from build123d import *

# Parameters (mm, degrees)
BOSS_EXTRUDE1_DEPTH = 6.35
CUT_EXTRUDE4_DEPTH  = 6.35
SKETCH3_R           = 3.2639
CUT_EXTRUDE5_DEPTH  = 6.35


with BuildPart() as part:
    # Sketch1 → Boss-Extrude1 (new body)
    with BuildSketch(Plane(origin=(0, 0, 0), x_dir=(0, 0, -1), z_dir=(1, 0, 0))):
        with BuildLine():
            Line((152.4, 0), (152.4, -50.8))
            Line((152.4, -50.8), (203.2, -50.8))
            Line((203.2, -50.8), (203.2, 0))
            ThreePointArc((203.2, 0), (190.945540544, 69.498493124), (155.660230842, 130.614442288))
            Line((155.660230842, 130.614442288), (116.745173131, 97.960831716))
            ThreePointArc((116.745173131, 97.960831716), (143.209155408, 52.123869843), (152.4, 0))
        make_face()
    extrude(amount=BOSS_EXTRUDE1_DEPTH)

    # Sketch2 → Cut-Extrude4 (cut)
    with BuildSketch(Plane(origin=(6.35, 0, 0), x_dir=(0, 0, -1), z_dir=(1, 0, 0))):
        with BuildLine():
            ThreePointArc((134.46138915, 101.323924376), (129.890458655, 101.966326764), (129.248056268, 97.395396268))
            ThreePointArc((129.248056268, 97.395396268), (153.473001896, 51.351348104), (161.8361, 0))
            ThreePointArc((161.8361, 0), (165.1, -3.2639), (168.3639, 0))
            ThreePointArc((168.3639, 0), (159.663469053, 53.422649441), (134.46138915, 101.323924376))
        make_face()
        with BuildLine():
            ThreePointArc((154.746731105, 116.610025965), (150.17580061, 117.252428352), (149.533398223, 112.681497856))
            ThreePointArc((149.533398223, 112.681497856), (177.560422739, 59.410886377), (187.2361, 0))
            ThreePointArc((187.2361, 0), (190.5, -3.2639), (193.7639, 0))
            ThreePointArc((193.7639, 0), (183.750889895, 61.482187713), (154.746731105, 116.610025965))
        make_face()
    extrude(amount=-CUT_EXTRUDE4_DEPTH, mode=Mode.SUBTRACT)

    # Sketch3 → Cut-Extrude5 (cut)
    with BuildSketch(Plane(origin=(6.35, 0, 0), x_dir=(0, 0, -1), z_dir=(1, 0, 0))):
        with Locations((165.1, -38.1)):
            Circle(SKETCH3_R)
        with Locations((190.5, -38.1)):
            Circle(SKETCH3_R)
    extrude(amount=-CUT_EXTRUDE5_DEPTH, mode=Mode.SUBTRACT)

    # Sketch7 → Cut-Revolve1 (revolve, cut)
    with BuildSketch(Plane(origin=(0, 0, 0), x_dir=(1, 0, 0), z_dir=(0, 1, 0))):
        with BuildLine():
            Line((-25.4, 38.1), (-144.027789746, 38.1))
            ThreePointArc((-144.027789746, 38.1), (-25.4, 156.727789746), (93.227789746, 38.1))
            Line((93.227789746, 38.1), (-25.4, 38.1))
        make_face()
    revolve(axis=Axis((-1000, 0, 0), (1, 0, 0)), mode=Mode.SUBTRACT)


solid = part.part
The model under review builds one solid part; all positions refer to its coordinate system, in mm. A direction names the side the tool comes from. Round coordinates to 2 decimals unless told otherwise and drop trailing zeros. Write each loop counter-clockwise with the first axis right and the second up, starting at its lowest first coordinate (ties: lowest second). Pieces come first, ordered by that corner, then holes. Notation, with made-up numbers: M 26,8 L 48,8 A8 cw 48,23 Z; hole C 16.5,-16.5 d8. An arc over 180 degrees is marked long. Use a Markdown table: item, result. Add a question column.
Q1. Insertion check: pin 1 (1.9 mm diameter, centred on x = 2.5, y = -33, fed in from +Z); pin 2 (5 mm diameter, centred on y = 32.5, z = -149, fed in from -X); pin 3 (3 mm diameter, centred on x = 0.5, z = -139, fed in from -Y); pin 4 (1 mm diameter, centred on x = 3, z = -137, fed in from +Y). Each pin has a flat end and moves straight along its axis. Give the tip position at first contact, or say it passes through.
Q2. We need section C-C, the plane z = -183. State the section outline as (x, y) points, plus the area to 3 significant figures.
Q3. We need section A-A, the plane y = -38.1. State the section outline as (x, z) points, plus the area to 3 significant figures.
Q4. To check wall thickness, follow line 1 (Z direction, x = 6, y = 88); line 2 (Z direction, x = 5.5, y = 56); line 3 (Z direction, x = 4.25, y = -28). State the ranges of each line that lie inside material, in increasing order.
Q5. We need section B-B, the plane z = -166. State the section outline as (x, y) points.
Q6. Machinability: for faces 5 (the face through (3.131, 68.565, -191.283)), 6 (the face through (3.219, -3.263, -190.428)), which of the approach directions +Z, -Z, +X, -X, +Y, -Y give a long, thin tool a straight path to every point of the face, cutting with its end or side? Answer none if there is none.
Q7. We need section D-D, the plane x = 4. Count the separate pieces of the cut face and the enclosed holes in it, plus the area to 3 significant figures.
Q8. The part is to be moulded in two halves that separate along Z. For faces 1 (the face through (3, -31, -152.4)), 2 (the face through (3.22, 60.21, -177.29)), 3 (the face through (3.22, 117.29, -150.23)), 4 (the face through (0, 41, -169)), say which applies: pulls with the +Z half, pulls with the -Z half, needs draft (parallel to the pull), parting line crosses it, or undercut.
Findings below:
| question | item | result |
|---|---|---|
| 1 | pin 1 | stops at z = -152.4 |
| 1 | pin 2 | stops at x = 0 |
| 1 | pin 3 | stops at y = 62.62 |
| 1 | pin 4 | stops at y = 115.38 |
| 2 | outline | M 0,-50.8 L 6.35,-50.8 L 6.35,39.6 L 0,39.6 Z; M 0,63.68 L 6.35,63.68 L 6.35,88.32 L 0,88.32 Z |
| 2 | area | 731 mm² |
| 3 | outline | M 0,-203.2 L 6.35,-203.2 L 6.35,-193.76 L 0,-193.76 Z; M 0,-187.24 L 6.35,-187.24 L 6.35,-168.36 L 0,-168.36 Z; M 0,-161.84 L 6.35,-161.84 L 6.35,-152.4 L 0,-152.4 Z |
| 3 | area | 240 mm² |
| 4 | line 1 | z = -183.16 to -172.63, -165.27 to -143.54, -135.82 to -124.54 |
| 4 | line 2 | z = -195.33 to -185.5, -178.67 to -158.78, -151.84 to -141.99 |
| 4 | line 3 | z = -203.2 to -152.4 |
| 5 | outline | M 0,-50.8 L 6.35,-50.8 L 6.35,-41.24 L 0,-41.24 Z; M 0,-34.96 L 6.35,-34.96 L 6.35,-3.14 L 0,-3.14 Z; M 0,28.11 L 6.35,28.11 L 6.35,86.61 L 0,86.61 Z; M 0,99.94 L 6.35,99.94 L 6.35,117.19 L 0,117.19 Z |
| 6 | face 5 | -Z, +X, -X, +Y |
| 6 | face 6 | +X, -X |
| 7 | separate pieces | 1 |
| 7 | enclosed holes | 4 |
| 7 | area | 7,180 mm² |
| 8 | face 1 | pulls with the +Z half |
| 8 | face 2 | undercut |
| 8 | face 3 | undercut |
| 8 | face 4 | needs draft |
